```python
from build123d import *

# Parameters (mm, degrees)
F1_DEPTH = 10
F2_DEPTH = 5


with BuildPart() as f1:
    # F0 (on Top) → F1 (new body)
    with BuildSketch(Plane.XY):
        with BuildLine():
            ThreePointArc((-44.218208919, -5), (-44.5, 0), (-44.218208919, 5))
            Line((-44.218208919, 5), (-54.5, 5))
            Line((-54.5, 5), (-54.5, -5))
            Line((-54.5, -5), (-44.218208919, -5))
        make_face()
        with BuildLine():
            Line((54.5, 5), (44.218208919, 5))
            ThreePointArc((44.218208919, 5), (44.4294963785, 2.503967163), (44.5, 0))
            ThreePointArc((44.5, 0), (44.4294963785, -2.503967163), (44.218208919, -5))
            Line((44.218208919, -5), (54.5, -5))
            Line((54.5, -5), (54.5, 5))
        make_face()
        with BuildLine():
            Line((42.5, -5), (42.5, 0))
            ThreePointArc((42.5, 0), (0, -42.5), (-42.5, 0))
            Line((-42.5, 0), (-42.5, -5))
            Line((-42.5, -5), (-44.218208919, -5))
            ThreePointArc((-44.218208919, -5), (-34.885846805, -27.626575841), (-15, -41.895703837))
            Line((-15, -41.895703837), (-12, -41.895703837))
            Line((-12, -41.895703837), (-12, -42.8514877221))
            ThreePointArc((-12, -42.8514877221), (0, -44.5), (12, -42.8514877221))
            Line((12, -42.8514877221), (12, -41.895703837))
            Line((12, -41.895703837), (15, -41.895703837))
            ThreePointArc((15, -41.895703837), (34.885846805, -27.626575841), (44.218208919, -5))
            Line((44.218208919, -5), (42.5, -5))
        make_face()
        with BuildLine():
            Line((42.5, 5), (42.5, 0))
            Line((42.5, 0), (42.5, -5))
            Line((42.5, -5), (44.218208919, -5))
            ThreePointArc((44.218208919, -5), (44.4294963785, -2.503967163), (44.5, 0))
            ThreePointArc((44.5, 0), (44.4294963785, 2.503967163), (44.218208919, 5))
            Line((44.218208919, 5), (42.5, 5))
        make_face()
        with BuildLine():
            ThreePointArc((-42.5, 0), (0, 42.5), (42.5, 0))
            Line((42.5, 0), (42.5, 5))
            Line((42.5, 5), (44.218208919, 5))
            ThreePointArc((44.218208919, 5), (0, 44.5), (-44.218208919, 5))
            Line((-44.218208919, 5), (-42.5, 5))
            Line((-42.5, 5), (-42.5, 0))
        make_face()
        with BuildLine():
            Line((-42.5, -5), (-42.5, 0))
            Line((-42.5, 0), (-42.5, 5))
            Line((-42.5, 5), (-44.218208919, 5))
            ThreePointArc((-44.218208919, 5), (-44.5, 0), (-44.218208919, -5))
            Line((-44.218208919, -5), (-42.5, -5))
        make_face()
        with BuildLine():
            Line((15, -51.895703837), (15, -41.895703837))
            ThreePointArc((15, -41.895703837), (13.5084558965, -42.4001370197), (12, -42.8514877221))
            Line((12, -42.8514877221), (12, -51.895703837))
            Line((12, -51.895703837), (15, -51.895703837))
        make_face()
        with BuildLine():
            ThreePointArc((-12, -42.8514877221), (-13.5084558965, -42.4001370197), (-15, -41.895703837))
            Line((-15, -41.895703837), (-15, -51.895703837))
            Line((-15, -51.895703837), (-12, -51.895703837))
            Line((-12, -51.895703837), (-12, -42.8514877221))
        make_face()
        with BuildLine():
            Line((-12, -41.895703837), (-15, -41.895703837))
            ThreePointArc((-15, -41.895703837), (-13.5084558965, -42.4001370197), (-12, -42.8514877221))
            Line((-12, -42.8514877221), (-12, -41.895703837))
        make_face()
        with BuildLine():
            ThreePointArc((12, -42.8514877221), (13.5084558965, -42.4001370197), (15, -41.895703837))
            Line((15, -41.895703837), (12, -41.895703837))
            Line((12, -41.895703837), (12, -42.8514877221))
        make_face()
    extrude(amount=F1_DEPTH)

    # F0 (on Top) → F2 (join)
    with BuildSketch(Plane.XY):
        with BuildLine():
            Line((12, -51.895703837), (12, -42.8514877221))
            ThreePointArc((12, -42.8514877221), (0, -44.5), (-12, -42.8514877221))
            Line((-12, -42.8514877221), (-12, -51.895703837))
            Line((-12, -51.895703837), (-15, -51.895703837))
            Line((-15, -51.895703837), (-15, -79.5))
            Line((-15, -79.5), (15, -79.5))
            Line((15, -79.5), (15, -51.895703837))
            Line((15, -51.895703837), (12, -51.895703837))
        make_face()
        with BuildLine():
            ThreePointArc((4.0721059777, -55.3666570793), (8.3881183759, -59.0557856295), (10, -64.5))
            ThreePointArc((10, -64.5), (-5.5100390097, -72.8450266693), (-3.9278940223, -55.303715503))
            Line((-3.9278940223, -55.303715503), (-3.9278940223, -49.5))
            Line((-3.9278940223, -49.5), (4.0721059777, -49.5))
            Line((4.0721059777, -49.5), (4.0721059777, -55.3666570793))
        make_face(mode=Mode.SUBTRACT)
    extrude(amount=F2_DEPTH)


solid = f1.part
```
Input: part model. Units: mm. Frame: model coordinates. A direction names the side the tool comes from. Round coordinates to 2 decimals unless told otherwise and drop trailing zeros. Loops run counter-clockwise (first coordinate to the right, second up) from the corner with the lowest first, then second, coordinate; pieces in that order, holes last.
1) Section query A-A on x = 0. Return the cut outline in (y, z), plus the area to 3 significant figures.
Ans:
outline: (-79.5, 0) - (-74.5, 0) - (-74.5, 5) - (-79.5, 5) - close; (-49.5, 0) - (-42.5, 0) - (-42.5, 10) - (-44.5, 10) - (-44.5, 5) - (-49.5, 5) - close; (42.5, 0) - (44.5, 0) - (44.5, 10) - (42.5, 10) - close
area: 90.0 mm2
2) Pull-direction query (Y, two-part tool) for faces 1 (the flat face through (0, -49.5, 2)), 2 (the flat face through (15, -57, 4)), 3 (the cylindrical face through (0.91, 44.49, 4.93)); classes: released by +Y, released by -Y, zero draft, split by the parting line, or undercut.
Ans:
face 1: undercut
face 2: zero draft
face 3: released by +Y
3) Material intervals for line 1 (X direction, y = -64.5, z = 3.35); line 2 (Y direction, x = 1, z = 3.5); line 3 (Y direction, x = 9.5, z = 8), sorted ascending.
Ans:
line 1: x = -15 to -10, 10 to 15
line 2: y = -79.5 to -74.45, -49.5 to -42.49, 42.49 to 44.49
line 3: y = -43.47 to -41.42, 41.42 to 43.47
4) Set-up query: faces 4 (the flat face through (-14, -51.896, 7)), 5 (the flat face through (4.072, -52, 2)), 6 (the flat face through (-49, 5, 5)). Return all of +Z, -Z, +X, -X, +Y, -Y with unobstructed straight access to the full face (end or side cutting, diameter ignored); none if empty.
Ans:
face 4: +Z, +X, -X, -Y
face 5: +Z, -Z
face 6: +Z, -Z, -X, +Y
5) Section query B-B on y = 0. Return the cut outline in (x, z), plus the area to 3 significant figures.
Ans:
outline: (-54.5, 0) - (-42.5, 0) - (-42.5, 10) - (-54.5, 10) - close; (42.5, 0) - (54.5, 0) - (54.5, 10) - (42.5, 10) - close
area: 240 mm2
6) Pin query (flat end, axial travel): pin 1 (3 mm diameter, centred on x = -52, z = 3.5, fed in from +Y); pin 2 (0.9 mm diameter, centred on x = 14, z = 8, fed in from -Y); pin 3 (4 mm diameter, centred on y = -47, z = 7.5, fed in from -X). Return the tip coordinate at first contact, or that it passes through.
Ans:
pin 1: stops at y = 5
pin 2: stops at y = -51.9
pin 3: stops at x = -15
7) Section query D-D on x = -26. Return the cut outline in (y, z).
Ans:
outline: (-36.11, 0) - (-33.62, 0) - (-33.62, 10) - (-36.11, 10) - close; (33.62, 0) - (36.11, 0) - (36.11, 10) - (33.62, 10) - close
8) Section query C-C on z = 7.5. Return the cut outline in (x, y), plus the area to 3 significant figures.
Ans:
outline: (-54.5, -5) - (-44.22, -5) arc R44.5 ccw to (-15, -41.9) - (-15, -51.9) - (-12, -51.9) - (-12, -42.85) arc R44.5 ccw to (12, -42.85) - (12, -51.9) - (15, -51.9) - (15, -41.9) arc R44.5 ccw to (44.22, -5) - (54.5, -5) - (54.5, 5) - (44.22, 5) arc R44.5 ccw to (-44.22, 5) - (-54.5, 5) - close; hole circle Ø85 at (0, 0)
area: 806 mm2
